Could you check a few things on this model? Use its own coordinates, in mm. A direction names the side the tool comes from. Coordinates: 2 decimals unless noted, no trailing zeros. Write each loop counter-clockwise with the first axis right and the second up, starting at its lowest first coordinate (ties: lowest second). Pieces come first, ordered by that corner, then holes. Notation, with made-up numbers: (-2, -12) - (6, -12) arc R23 cw to (6, 15) - close; hole circle Ø10 at (38.25, 29). An arc over 180 degrees is marked (long way). Answer as a JSON object with one key per item and string values. Group by question number.
1) Will these pins go through, and if not, where does the flat tip stop? pin 1 Ø8 at (y, z) = (8, 8.5) entering from -X; pin 2 Ø10 at (y, z) = (-11, 1.5) entering from -X; pin 3 Ø1.1 at (y, z) = (-1, -11) entering from +X.
2) On a 3-axis mill with a long thin cutter (end or side, diameter ignored), from which of +Z, -Z, +X, -X, +Y, -Y can I reach the whole of each face in a straight line? I mean faces 4 (the flat face through (59, 0, 11.25)), 5 (the flat face through (20, 0, 10.25)), 6 (the flat face through (19.428, 4.918, -10.757)). Say none if no direction works.
3) Please list where these lines run through material, in increasing order: line 1 along Y through (x, z) = (0, 6.5); line 2 along X through (y, z) = (0.5, 7.75); line 3 along X through (y, z) = (-1.5, -0.5).
4) If we section it at A-A (z = 5): Write out the boundary of the cut face in (x, y), plus the area to 3 significant figures.
5) We'd pull the mould along Y, two halves only. Please class faces 1 (the flat face through (100, 0, 10.25)), 2 (the cylindrical face through (-14.496, 0.346, 0.116)), 3 (the flat face through (59, 0, -11.25)): released by +Y, released by -Y, zero draft, split by the parting line, or undercut.
```python
from build123d import *

# Parameters (mm, degrees)
BOSS_EXTRU_1_DEPTH      = 11.25
CONG_1_R                = 3
CONG_1_OF_SYM_TRIE5_R   = 3
ENL_V_MAT_EXTRU_1_DEPTH = 1


with BuildPart() as part:
    # Esquisse1 → Boss.-Extru.1 (new body)
    with BuildSketch(Plane.XY):
        with BuildLine():
            ThreePointArc((1.924778761, 14.371681416), (-9.548316814, 10.912362073), (-14.5, 0))
            Line((-14.5, 0), (-4, 0))
            ThreePointArc((-4, 0), (0, 4), (4, 0))
            Line((4, 0), (116, 0))
            ThreePointArc((116, 0), (120, 4), (124, 0))
            Line((124, 0), (134.5, 0))
            ThreePointArc((134.5, 0), (129.548316814, 10.912362073), (118.075221239, 14.371681416))
            ThreePointArc((118.075221239, 14.371681416), (60, 10.5), (1.924778761, 14.371681416))
        make_face()
        with BuildLine():
            Line((-4, 0), (-14.5, 0))
            ThreePointArc((-14.5, 0), (-9.548316814, -10.912362073), (1.924778761, -14.371681416))
            ThreePointArc((1.924778761, -14.371681416), (60, -10.5), (118.075221239, -14.371681416))
            ThreePointArc((118.075221239, -14.371681416), (129.548316814, -10.912362073), (134.5, 0))
            Line((134.5, 0), (124, 0))
            ThreePointArc((124, 0), (120, -4), (116, 0))
            Line((116, 0), (4, 0))
            ThreePointArc((4, 0), (0, -4), (-4, 0))
        make_face()
    boss_extru_1 = extrude(amount=BOSS_EXTRU_1_DEPTH)

    # Cong_1
    cong_1_edges = [part.edges().sort_by_distance(p)[0] for p in [
        (-14.5, 0, 11.25),
        (60, -10.5, 11.25),
        (134.5, 0, 11.25),
        (60, 10.5, 11.25),
    ]]
    fillet(cong_1_edges, radius=CONG_1_R)

    # Sym_trie5: Boss.-Extru.1 across plane
    add(boss_extru_1.mirror(Plane.XY))

    # Cong_1 of Sym_trie5
    cong_1_of_sym_trie5_edges = [part.edges().sort_by_distance(p)[0] for p in [
        (-14.5, 0, -11.25),
        (60, -10.5, -11.25),
        (134.5, 0, -11.25),
        (60, 10.5, -11.25),
    ]]
    fillet(cong_1_of_sym_trie5_edges, radius=CONG_1_OF_SYM_TRIE5_R)

    # Esquisse3 → Enl_v. mat.-Extru.1 (cut)
    with BuildSketch(Plane.XY.offset(11.25)):
        with BuildLine():
            Line((10.5, 6.782329983), (28.609223614, 3))
            Line((28.609223614, 3), (28.609223614, -3))
            Line((28.609223614, -3), (10.5, -6.782329983))
            ThreePointArc((10.5, -6.782329983), (12.5, 0), (10.5, 6.782329983))
        make_face()
        with BuildLine():
            Line((91.390776386, -3), (109.5, -6.782329983))
            ThreePointArc((109.5, -6.782329983), (107.5, 0), (109.5, 6.782329983))
            Line((109.5, 6.782329983), (91.390776386, 3))
            Line((91.390776386, 3), (91.390776386, -3))
        make_face()
    enl_v_mat_extru_1 = extrude(amount=-ENL_V_MAT_EXTRU_1_DEPTH, mode=Mode.SUBTRACT)

    # Sym_trie6: Enl_v. mat.-Extru.1 across plane
    add(enl_v_mat_extru_1.mirror(Plane.XY), mode=Mode.SUBTRACT)


solid = part.part
```
Here are the results:
{
 "1": {"pin 1": "stops at x = -13.94", "pin 2": "stops at x = -13.2", "pin 3": "stops at x = 133.5"},
 "2": {"face 4": "+Z, +X, -X, +Y, -Y", "face 5": "+Z", "face 6": "-Z"},
 "3": {"line 1": "y = -14.5 to -4, 4 to 14.5", "line 2": "x = -14.49 to -3.97, 3.97 to 116.03, 123.97 to 134.49", "line 3": "x = -14.42 to -3.71, 3.71 to 116.29, 123.71 to 134.42"},
 "4": {"outline": "(1.92, -14.37) arc R437.5 cw to (118.08, -14.37) arc R14.5 ccw (long way) to (118.08, 14.37) arc R437.5 cw to (1.92, 14.37) arc R14.5 ccw (long way) to start; hole circle Ø8 at (0, 0); hole circle Ø8 at (120, 0)", "area": "3,410 mm²"},
 "5": {"face 1": "undercut", "face 2": "split by the parting line", "face 3": "zero draft"}
}
